The model under review builds one solid part; all positions refer to its coordinate system, in mm. Face numbers are marked on the shaded views. A direction names the side the tool comes from. Coordinates: 2 decimals unless noted, no trailing zeros. Write each loop counter-clockwise with the first axis right and the second up, starting at its lowest first coordinate (ties: lowest second). Pieces come first, ordered by that corner, then holes. Notation, with made-up numbers: (68, -3.75) - (109, -3.75) arc R18 cw to (109, 11.25) - close; hole circle Ø4 at (45, -4.75). An arc over 180 degrees is marked (long way). Return JSON: item names as keys, results as strings. Group by question number.
(1) For pin 1 Ø3.5 at (y, z) = (42.5, 12.5) entering from +X; pin 2 Ø3 at (x, y) = (17, 15) entering from +Z; pin 3 Ø1 at (x, y) = (53.5, 82) entering from -Z; pin 4 Ø7.5 at (y, z) = (17.5, 10) entering from +X, all flat-tipped, find the tip position at first contact; note any pin that passes through.
(2) We need section A-A on y = 7.5. State the section outline as (x, z) points, then the cut area to 3 significant figures.
(3) We need section C-C on y = 22.5. State the section outline as (x, z) points, then the cut area to 3 significant figures.
(4) We need section B-B on x = 52.5. State the section outline as (y, z) points, then the cut area to 3 significant figures.
(5) Tool access review of the marked faces 1 and 2: name each direction out of +Z, -Z, +X, -X, +Y, -Y from which nothing blocks a thin tool from reaching the whole face with its end or side.
(6) We need section D-D on z = 12.25. State the section outline as (x, y) points.
(7) To check wall thickness, follow L1, parallel to Y at x = 52.5, z = 1.2; L2, parallel to Y at x = 1.1, z = 12.5; L3, parallel to X at y = 20, z = 14.25. State the ranges of each line that lie inside material, in increasing order. Write a range as from..to.
Autodesk Inventor part; units mm, degrees
ref_plane "YZ Plane" through (0, 0, 0) normal (1, 0, 0) x (0, 1, 0)
ref_plane "XZ Plane" through (0, 0, 0) normal (0, 1, 0) x (-1, 0, 0)
ref_plane "XY Plane" through (0, 0, 0) normal (0, 0, 1) x (1, 0, 0)
sketch "Sketch1" plane through (0, 0, 0) normal (0, 0, 1) x (1, 0, 0)
  line L0 (0, 0) -> (65, 0)
  line L1 (65, 0) -> (65, 102)
  line L2 (65, 102) -> (0, 102)
  line L3 (0, 102) -> (0, 0)
  line L4 (0, 50) -> (5, 50)
  line L5 (5, 50) -> (57, 102)
  dimension "d0" = 65
  dimension "d1" = 102
  dimension "d28" = 45
  dimension "d29" = 50
  dimension "d30" = 5
extrude "Extrusion1" add sketch "Sketch1" along normal blind 3 contours L3 L4 L5 L2 L1 L0
sketch "Sketch2" plane through (0, 0, 3) normal (0, 0, 1) x (1, 0, 0)
  line L0 (0, 0) -> (65, 0)
  line L1 (0, 0) -> (3, 0)
  line L2 (3, 0) -> (3, 50)
  line L3 (3, 50) -> (0, 50)
  line L4 (0, 50) -> (0, 0)
  dimension "d4" = 3
  dimension "d5" = 50
extrude "Extrusion2" add sketch "Sketch2" along normal blind 17
chamfer "Chamfer2" distance 45 angle 45 1 edges at (65, 0, 1.5)
sketch "Sketch4" plane through (3, 0, 3) normal (1, 0, 0) x (0, 0, -1)
  line L0 (-17, 0) -> (-17, 50)
  line L1 (0, 50) -> (-17, 50)
  line L2 (0, 0) -> (-17, 0)
  point P0 (3, 0)
  point P1 (-9.5, 42.5)
  point P2 (-9.5, 7.5)
  dimension "d31" = 7.5
  dimension "d32" = 7.5
  dimension "d33" = 7.5
  dimension "d34" = 35
hole "Hole1" at (3, 42.5, 12.5) at (3, 7.5, 12.5) direction (-1, 0, 0) diameter 4.5 end through all
sketch "Sketch3" plane through (0, 0, 3) normal (0, 0, 1) x (1, 0, 0)
  line L0 (3, 0) -> (3, 50)
  line L1 (0, 50) -> (0, 0)
  line L2 (3, 50) -> (0, 50)
  point P0 (57.5, 95)
  dimension "d10" = 57.5
  dimension "d42" = 45
hole "Hole2" at (57.5, 95, 3) direction (0, 0, -1) diameter 6 end through all
sketch "Sketch5" plane through (0, 0, 3) normal (0, 0, 1) x (1, 0, 0)
  circle A0 centre (57.5, 95) radius 3
  point P0 (0, 0)
  point P1 (52.5, 71)
  point P2 (52.5, 49)
  dimension "d51" = 22
  dimension "d70" = 24
  dimension "d71" = 5
hole "Hole3" at (52.5, 71, 3) at (52.5, 49, 3) direction (0, 0, -1) diameter 3.4 end through all
fillet "Fillet5" radius 2 1 edges at (3, 25, 3)
fillet "Fillet6" radius 5 1 edges at (0, 25, 0)
sketch "Sketch6" plane through (0, 0, 3) normal (0, 0, 1) x (1, 0, 0)
  circle A0 centre (57.5, 95) radius 3
  circle A1 centre (52.5, 71) radius 1.7
  point P0 (0, 0)
  point P1 (52.5, 60)
  dimension "d69" = 11
hole "Hole4" at (52.5, 60, 3) direction (0, 0, -1) diameter 8 end through all
properties part number "Pancake_Bracket" material "Aluminum 6061"
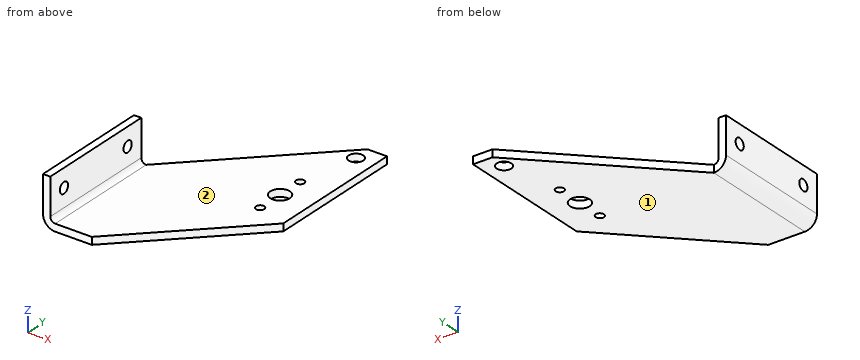
Ans:
{
 "1": {"pin 1": "through", "pin 2": "z = 3", "pin 3": "z = 0", "pin 4": "x = 3"},
 "2": {"outline": "(0, 5) arc R5 ccw to (5, 0) - (27.5, 0) - (27.5, 3) - (5, 3) arc R2 cw to (3, 5) - (3, 10.25) - (0, 10.25) - close; (0, 14.75) - (3, 14.75) - (3, 20) - (0, 20) - close", "area": "115 mm²"},
 "3": {"outline": "(0, 5) arc R5 ccw to (5, 0) - (42.5, 0) - (42.5, 3) - (5, 3) arc R2 cw to (3, 5) - (3, 20) - (0, 20) - close", "area": "174 mm²"},
 "4": {"outline": "(32.5, 0) - (47.3, 0) - (47.3, 3) - (32.5, 3) - close; (50.7, 0) - (56, 0) - (56, 3) - (50.7, 3) - close; (64, 0) - (69.3, 0) - (69.3, 3) - (64, 3) - close; (72.7, 0) - (97.5, 0) - (97.5, 3) - (72.7, 3) - close", "area": "151 mm²"},
 "5": {"face 1": "-Z, +X, -X, +Y, -Y", "face 2": "+Z, +X, +Y, -Y"},
 "6": {"outline": "(0, 0) - (3, 0) - (3, 5.26) - (0, 5.26) - close; (0, 9.74) - (3, 9.74) - (3, 40.26) - (0, 40.26) - close; (0, 44.74) - (3, 44.74) - (3, 50) - (0, 50) - close"},
 "7": {"L1": "32.5..47.3, 50.7..56, 64..69.3, 72.7..97.5", "L2": "0..5.25, 9.75..40.25, 44.75..50", "L3": "0..3"}
}
